Read the model definition and answer for the solid it produces. Units are mm, in the model's axes. A direction names the side the tool comes from. Give positions to 0.01 mm unless a question says otherwise; leave off trailing zeros. Loops run counter-clockwise (first coordinate to the right, second up) from the corner with the lowest first, then second, coordinate; pieces in that order, holes last. Notation, with made-up numbers: (57, 33) -> (100, 33) arc R35 ccw to (100, 71) -> close; hole circle Ø7 at (61.25, 29). An arc over 180 degrees is marked (long way). Write each question's results on one line, items separated by ' | '. Start each with the question number.
Item 1: Section D-D on y = 98 is taken. Write down the section's boundary in (x, z), and give its area (4 significant figures).
Item 2: Find the intervals of material crossed by line 1 (X direction, y = 18, z = 81); line 2 (Y direction, x = 2, z = 24); line 3 (Y direction, x = 8, z = 30), in increasing order.
Item 3: Each of these flat-tipped pins is pushed along its axis until it touches: P1, Ø1.1, axis at x = 5, y = 259, coming from the +Z side; P2, Ø3, axis at x = 5, y = 17.5, coming from the -Z side. Where does it stop, or does it pass through?
Item 4: Which of the six approach directions +Z, -Z, +X, -X, +Y, -Y give full straight-line access (tool end or side, diameter ignored) to faces 1 (the flat face through (6, 218, 20)), 2 (the cylindrical face through (6, 181, 79)), 3 (the cylindrical face through (5.35, 15.07, 77.14))?
Item 5: Section A-A on y = 243 is taken. Write down the section's boundary in (x, z), and give its area (3 significant figures).
Item 6: Section C-C on z = 30 is taken. Write down the section's boundary in (x, y).
Item 7: Section B-B on z = 11.5 is taken. Write down the section's boundary in (x, y).
Item 8: Determine the mould class of faces 4 (the flat face through (6, 0, 43)), 5 (the flat face through (12, 136, 44)), 6 (the flat face through (6, 58, 67)) for opening direction Y: +Y half, -Y half, draft (parallel to the pull), parting line (faces both ways), or undercut.
```python
from build123d import *

# Parameters (mm, degrees)
F0_W     = 276
F0_H     = 87
F1_DEPTH = 12
F2_R     = 27.5
F3_DEPTH = 25
F4_R     = 3
F5_DEPTH = 20
F6_R     = 3
F7_DEPTH = 20


with BuildPart() as f1:
    # F0 (on Right) → F1 (new body)
    with BuildSketch(Plane.YZ):
        with Locations((138, 43.5)):
            Rectangle(F0_W, F0_H)
    extrude(amount=F1_DEPTH)

    # F2 (on face) → F3 (cut)
    with BuildSketch(Plane.YZ.offset(12)):
        with Locations((103, 43.5)):
            Circle(F2_R)
        with Locations((173, 43.5)):
            Circle(F2_R)
        with Locations((33, 43.5)):
            Circle(F2_R)
        with Locations((243, 43.5)):
            Circle(F2_R)
    extrude(amount=-F3_DEPTH, mode=Mode.SUBTRACT)

    # F4 (on face) → F5 (cut)
    with BuildSketch(Plane.XY.offset(87)):
        with Locations((6, 258)):
            Circle(F4_R)
        with Locations((6, 218)):
            Circle(F4_R)
        with Locations((6, 178)):
            Circle(F4_R)
        with Locations((6, 18)):
            Circle(F4_R)
        with Locations((6, 58)):
            Circle(F4_R)
        with Locations((6, 98)):
            Circle(F4_R)
    extrude(amount=-F5_DEPTH, mode=Mode.SUBTRACT)

    # F6 (on face) → F7 (cut)
    with BuildSketch(Plane(origin=(0, 0, 0), x_dir=(1, 0, 0), z_dir=(0, 0, -1))):
        with BuildLine():
            ThreePointArc((6, -255), (3, -258), (6, -261))
            Line((6, -261), (6, -258))
            Line((6, -258), (6, -255))
        make_face()
        with BuildLine():
            ThreePointArc((6, -175), (3, -178), (6, -181))
            Line((6, -181), (6, -175))
        make_face()
        with BuildLine():
            Line((6, -175), (6, -181))
            ThreePointArc((6, -181), (8.12132, -180.12132), (9, -178))
            ThreePointArc((9, -178), (8.12132, -175.87868), (6, -175))
        make_face()
        with BuildLine():
            ThreePointArc((6, -215), (3, -218), (6, -221))
            Line((6, -221), (6, -218))
            Line((6, -218), (6, -215))
        make_face()
        with BuildLine():
            Line((6, -218), (6, -221))
            ThreePointArc((6, -221), (8.12132, -220.12132), (9, -218))
            ThreePointArc((9, -218), (8.12132, -215.87868), (6, -215))
            Line((6, -215), (6, -218))
        make_face()
        with BuildLine():
            Line((6, -258), (6, -261))
            ThreePointArc((6, -261), (8.12132, -260.12132), (9, -258))
            Line((9, -258), (6, -258))
        make_face()
        with BuildLine():
            Line((6, -255), (6, -258))
            Line((6, -258), (9, -258))
            ThreePointArc((9, -258), (8.12132, -255.87868), (6, -255))
        make_face()
        with BuildLine():
            Line((6, -18), (9, -18))
            ThreePointArc((9, -18), (3.87868, -15.87868), (6, -21))
            Line((6, -21), (6, -18))
        make_face()
        with BuildLine():
            ThreePointArc((9, -58), (8.12132, -55.87868), (6, -55))
            ThreePointArc((6, -55), (3.87868, -60.12132), (9, -58))
        make_face()
        with BuildLine():
            ThreePointArc((6, -21), (8.12132, -20.12132), (9, -18))
            Line((9, -18), (6, -18))
            Line((6, -18), (6, -21))
        make_face()
        with Locations((6, -98)):
            Circle(F6_R)
    extrude(amount=-F7_DEPTH, mode=Mode.SUBTRACT)


solid = f1.part
```
Findings:
1) outline: (0, 0) -> (3, 0) -> (3, 16.46) -> (0, 16.46) -> close; (0, 70.54) -> (3, 70.54) -> (3, 87) -> (0, 87) -> close; (9, 0) -> (12, 0) -> (12, 16.46) -> (9, 16.46) -> close; (9, 70.54) -> (12, 70.54) -> (12, 87) -> (9, 87) -> close | area: 197.5 mm2
2) line 1: 0 to 3, 9 to 12 | line 2: 0 to 13.61, 52.39 to 83.61, 122.39 to 153.61, 192.39 to 223.61, 262.39 to 276 | line 3: 0 to 9.04, 56.96 to 79.04, 126.96 to 149.04, 196.96 to 219.04, 266.96 to 276
3) P1: z = 67 | P2: z = 20
4) face 1: -Z | face 2: +Z, -Z | face 3: +Z
5) outline: (0, 0) -> (12, 0) -> (12, 16) -> (0, 16) -> close; (0, 71) -> (12, 71) -> (12, 87) -> (0, 87) -> close | area: 384 mm2
6) outline: (0, 0) -> (12, 0) -> (12, 9.04) -> (0, 9.04) -> close; (0, 56.96) -> (12, 56.96) -> (12, 79.04) -> (0, 79.04) -> close; (0, 126.96) -> (12, 126.96) -> (12, 149.04) -> (0, 149.04) -> close; (0, 196.96) -> (12, 196.96) -> (12, 219.04) -> (0, 219.04) -> close; (0, 266.96) -> (12, 266.96) -> (12, 276) -> (0, 276) -> close
7) outline: (0, 0) -> (12, 0) -> (12, 276) -> (0, 276) -> close; hole circle Ø6 at (6, 98); hole (6, 21) arc R3 ccw (long way) to (9, 18) arc R3 ccw to start; hole (6, 55) arc R3 ccw to (9, 58) arc R3 ccw (long way) to start; hole (6, 175) arc R3 ccw to (9, 178) arc R3 ccw to (6, 181) arc R3 ccw to start; hole (6, 215) arc R3 ccw to (9, 218) arc R3 ccw to (6, 221) arc R3 ccw to start; hole (6, 255) arc R3 ccw to (9, 258) arc R3 ccw to (6, 261) arc R3 ccw to start
8) face 4: -Y half | face 5: draft | face 6: undercut
